Study the drawing (mm; zero at the part's minimum x, y, z) and answer. Round coordinates to 2 decimals unless told otherwise and drop trailing zeros. Write each loop counter-clockwise with the first axis right and the second up, starting at its lowest first coordinate (ties: lowest second). Pieces come first, ordered by that corner, then holes.
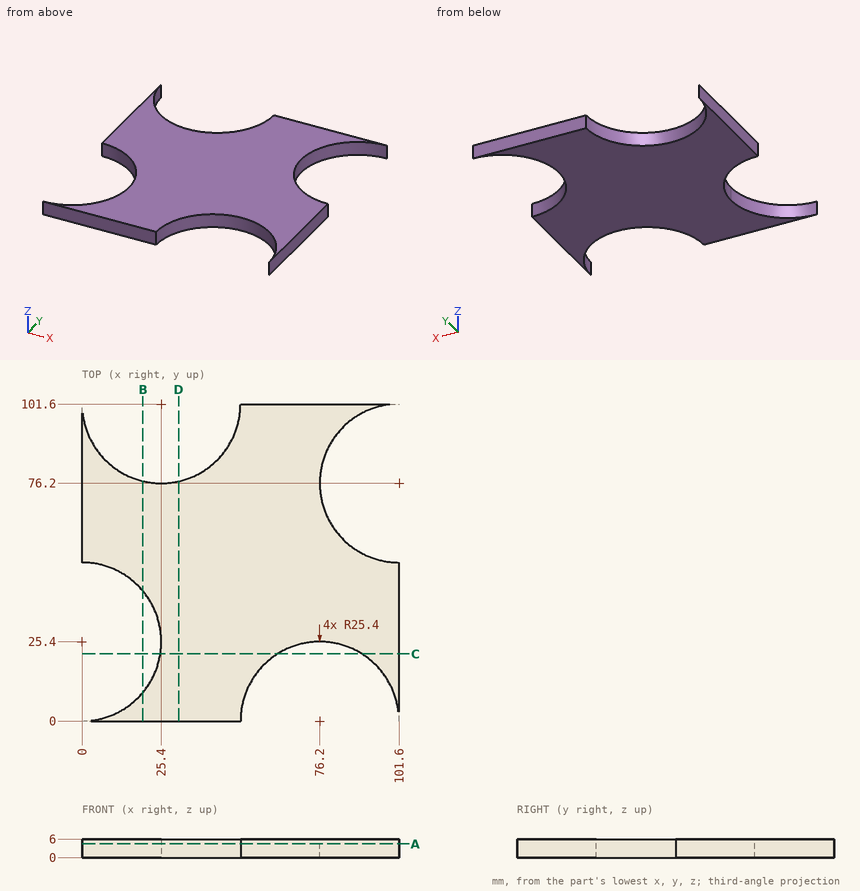
1. Given pin 1 (1 mm diameter, centred on x = 73, z = 3.5, fed in from -Y); pin 2 (1 mm diameter, centred on y = 52.5, z = 3, fed in from -X), each flat-ended and moving along its own axis, determine where each tip first touches the part or whether it passes through.
Geometry says:
pin 1: stops at y = 25.13
pin 2: stops at x = 0
2. Section B-B on x = 19.5 is taken. Determine the outline of the cut face in (y, z).
Geometry says:
outline: (0, 0) - (9.12, 0) - (9.12, 6) - (0, 6) - close; (41.68, 0) - (76.89, 0) - (76.89, 6) - (41.68, 6) - close
3. Section D-D on x = 31 is taken. Determine the outline of the cut face in (y, z), plus the area to 3 significant figures.
Geometry says:
outline: (0, 0) - (76.83, 0) - (76.83, 6) - (0, 6) - close
area: 461 mm2
4. Section C-C on y = 21.5 is taken. Determine the outline of the cut face in (x, z).
Geometry says:
outline: (25.1, 0) - (62.68, 0) - (62.68, 6) - (25.1, 6) - close; (89.72, 0) - (101.6, 0) - (101.6, 6) - (89.72, 6) - close
5. Straight lines are drawn through the part: line 1 along Y through (x, z) = (80, 4.3); line 2 along Y through (x, z) = (8, 4.2); line 3 along X through (y, z) = (13.5, 0.8). For each, find the intervals that lie inside material, in ascending order.
Geometry says:
line 1: y = 25.11 to 62.84, 89.56 to 101.6
line 2: y = 0 to 1.29, 49.51 to 83.1
line 3: x = 22.44 to 54.68, 97.72 to 101.6
6. Section A-A on z = 4.4 is taken. Determine the outline of the cut face in (x, y).
Geometry says:
outline: (0, 0) - (50.8, 0) arc R25.4 cw to (101.6, 0) - (101.6, 50.8) arc R25.4 cw to (101.6, 101.6) - (50.8, 101.6) arc R25.4 cw to (0, 101.6) - (0, 50.8) arc R25.4 cw to start
